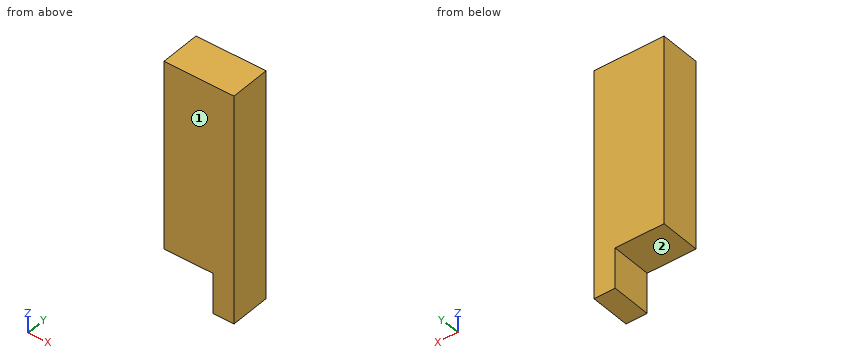
```python
from build123d import *

# Parameters (mm, degrees)
SKETCH1_W           = 33.02
SKETCH1_H           = 88.9
BOSS_EXTRUDE1_DEPTH = 9.525
SKETCH2_W           = 10
SKETCH2_H           = 19.05
BOSS_EXTRUDE2_DEPTH = 19.05


with BuildPart() as part:
    # Sketch1 → Boss-Extrude1 (new body, symmetric)
    with BuildSketch(Plane(origin=(0, 0, 0), x_dir=(1, 0, 0), z_dir=(0, 1, 0))):
        Rectangle(SKETCH1_W, SKETCH1_H)
    extrude(amount=BOSS_EXTRUDE1_DEPTH, both=True)

    # Sketch2 → Boss-Extrude2 (add)
    with BuildSketch(Plane(origin=(0, 0, -44.45), x_dir=(-1, 0, 0), z_dir=(0, 0, -1))):
        with Locations((-11.51, 0)):
            Rectangle(SKETCH2_W, SKETCH2_H)
    extrude(amount=BOSS_EXTRUDE2_DEPTH)


solid = part.part
```
Can you work these out from the model? Positions are in its coordinate system, mm. Face numbers are marked on the shaded views. A direction names the side the tool comes from. Coordinates: 2 decimals unless noted, no trailing zeros. Order: outer loops, then holes, each group sorted by start corner. A loop starts at its lowest first (then second) coordinate and runs counter-clockwise, first axis right, second up. Notation, with made-up numbers: (-39.75, -28) -> (9.25, -28) arc R9 ccw to (9.25, -23) -> close; hole circle Ø4 at (-40, -3). An arc over 180 degrees is marked (long way). Write each question's results on one line, items separated by ' | '.
Item 1: I'm going to push flat-ended pins straight in: pin 1 Ø5.5 at (x, y) = (-0.5, 0.5) entering from -Z; pin 2 Ø5.5 at (y, z) = (-2.5, -55) entering from -X. Where does each tip first touch, or does it pass through?
Results are:
pin 1: z = -44.45 | pin 2: x = 6.51
Item 2: If I drill on line 1 along Z through (x, y) = (-9, -8); line 2 along X through (y, z) = (4.75, -48), over which ranges is the centre line in solid material (lowest first)?
Results are:
line 1: -44.45 to 44.45 | line 2: 6.51 to 16.51
Item 3: I want a section at C-C, the plane x = -7.5. Write out the boundary of the cut face in (y, z) (3 decimals).
Results are:
outline: (-9.525, -44.45) -> (9.525, -44.45) -> (9.525, 44.45) -> (-9.525, 44.45) -> close
Item 4: I want a section at A-A, the plane y = -6.75. Write out the boundary of the cut face in (x, z), then the cut area to 3 significant figures.
Results are:
outline: (-16.51, -44.45) -> (6.51, -44.45) -> (6.51, -63.5) -> (16.51, -63.5) -> (16.51, 44.45) -> (-16.51, 44.45) -> close | area: 3,130 mm²
Item 5: I want a section at B-B, the plane z = -46.5. Write out the boundary of the cut face in (x, y) (3 decimals), then the cut area to 4 significant figures.
Results are:
outline: (6.51, -9.525) -> (16.51, -9.525) -> (16.51, 9.525) -> (6.51, 9.525) -> close | area: 190.5 mm²
Item 6: Which directions (+Z, -Z, +X, -X, +Y, -Y) give clear straight access to the entire face, cutting with the end or side of a thin tool? Please do the marked faces 1 and 2.
Results are:
face 1: +Z, -Z, +X, -X, -Y | face 2: -Z, -X, +Y, -Y
